from build123d import *

# Parameters (mm, degrees)
SKETCH_2_R          = 6
SKETCH_2_R_2        = 2.5
CUT_EXTRUDE_1_DEPTH = 0.7
CUT_EXTRUDE_START   = 0.7
SKETCH_3_R          = 6
SKETCH_3_R_2        = 2.5
CUT_EXTRUDE_2_DEPTH = 0.7


with BuildPart() as part:
    # ｽｹｯﾁ1 → 回転1 (revolve)
    with BuildSketch(Plane.XY, mode=Mode.PRIVATE) as revolve_1_sk:
        Polygon((0, 0), (0, 2.5), (0.5, 3), (61.5, 3), (62, 2.5), (62, 0), align=None)
    revolve(revolve_1_sk.sketch.rotate(Axis((62, 0, 0), (-1, 0, 0)), 270), axis=Axis((62, 0, 0), (-1, 0, 0)))

    # ｽｹｯﾁ2 → ｶｯﾄ - 押し出し1 (cut)
    with BuildSketch(Plane(origin=(5, 0, 0), x_dir=(0, 0, -1), z_dir=(1, 0, 0))):
        Circle(SKETCH_2_R)
        Circle(SKETCH_2_R_2, mode=Mode.SUBTRACT)
    extrude(amount=-CUT_EXTRUDE_1_DEPTH, mode=Mode.SUBTRACT)

    # ｽｹｯﾁ3 → ｶｯﾄ - 押し出し2 (cut)
    with BuildSketch(Plane(origin=(57, 0, 0), x_dir=(0, 0, -1), z_dir=(1, 0, 0)).offset(CUT_EXTRUDE_START)):
        Circle(SKETCH_3_R)
        Circle(SKETCH_3_R_2, mode=Mode.SUBTRACT)
    extrude(amount=-CUT_EXTRUDE_2_DEPTH, mode=Mode.SUBTRACT)


solid = part.part
Model file for the job. Use its own axes, mm. A direction names the side the tool comes from. Round coordinates to 2 decimals unless told otherwise and drop trailing zeros. Order: outer loops, then holes, each group sorted by start corner. A loop starts at its lowest first (then second) coordinate and runs counter-clockwise, first axis right, second up.
(1) Drill centre lines: line 1 (X direction, y = -0.8, z = -2.6); line 2 (X direction, y = -1.8, z = -1.85); line 3 (Z direction, x = 21.5, y = -0.25). Where is each one in solid material? Low to high.
(2) 3-axis set-ups, long thin cutter, end or side, ignore diameter. For faces 1 (the face through (4.3, 2, 2)), 2 (the face through (59.63, 0.9, 2.86)): which of +Z, -Z, +X, -X, +Y, -Y reach the whole face in a straight line?
(3) Pin check, flat tip, straight feed: pin 1 (3 mm diameter, centred on x = 46, z = -2, fed in from +Y). Stop position of the tip, or through.
(4) Band-saw the part on A-A (x = 53.5). List the corners of the cut face in (y, z).
Verdict:
1. line 1: x = 0.22 to 4.3, 5 to 57, 57.7 to 61.78
1. line 2: x = 0.08 to 4.3, 5 to 57, 57.7 to 61.92
1. line 3: z = -2.99 to 2.99
2. face 1: none
2. face 2: +X, -X
3. pin 1: stops at y = 2.96
4. outline: circle Ø6 at (0, 0)
